The listing builds one solid part. Answer for the finished solid, in the listing's coordinates (mm). A direction names the side the tool comes from. Round coordinates to 2 decimals unless told otherwise and drop trailing zeros. Write each loop counter-clockwise with the first axis right and the second up, starting at its lowest first coordinate (ties: lowest second). Pieces come first, ordered by that corner, then holes. Notation, with made-up numbers: M 25,50.5 L 37,50.5 A12 ccw 37,59.5 Z; hole C 4,8.5 d9. An arc over 180 degrees is marked long. One line per item, written item: value. Start each with the question number.
(1) Given P1, Ø3, axis at x = -14, y = 0.5, coming from the +Z side; P2, Ø1.5, axis at x = 7.5, y = 2, coming from the -Z side; P3, Ø0.5, axis at x = -15, z = 0.5, coming from the -Y side, each flat-ended and moving along its own axis, determine where each tip first touches the part or whether it passes through.
(2) Section A-A (z = 0.6) is taken. Determine the outline of the cut face in (x, y) (3 decimals), plus the area to 3 significant figures.
(3) For a pull along X with two mould halves and no side action, classify faces 1 (the flat face through (0, -7, 1.092)), 2 (the flat face through (16.835, 7.3, 0.6)), 3 (the flat face through (9.835, 7.3, 0.6)) as released by +X, released by -X, zero draft, split by the parting line, or undercut.
(4) Consider probe 1 along X at (y, z) = (-8.5, 0.6); probe 2 along Y at (x, z) = (-14.5, 0.95) (3 decimals). Determine where each line is inside the solid, lowest interval first.
(5) Section C-C (x = 2.5) is taken. Determine the outline of the cut face in (y, z) (3 decimals).
(6) Section B-B (y = 7.5) is taken. Determine the outline of the cut face in (x, z).
(7) For faces 4 (the flat face through (-13.4, -5.123, 0.6)), 5 (the flat face through (-13.4, 9.525, 0.6)), 6 (the flat face through (13.3, -9.523, 0.6)), determine the directions among +Z, -Z, +X, -X, +Y, -Y from which every point of the face is accessible in a straight line to the end or side of a thin tool.
(8) Section D-D (x = 7) is taken. Determine the outline of the cut face in (y, z).
```python
from build123d import *

# Parameters (mm, degrees)
F0_W     = 41.0972
F0_H     = 25.4
F1_DEPTH = 0.0762
F2_W     = 7
F2_H     = 4.4
F3_DEPTH = 1.016
F4_DEPTH = 0.2032


with BuildPart() as f1:
    # F0 (on Top) → F1 (new body)
    with BuildSketch(Plane.XY):
        Rectangle(F0_W, F0_H)
    extrude(amount=F1_DEPTH)

    # F2 (on face) → F3 (join)
    with BuildSketch(Plane.XY.offset(0.0762)):
        with Locations((-13.33512, 7.325)):
            Rectangle(F2_W, F2_H)
        with Locations((-13.33512, -7.32318)):
            Rectangle(F2_W, F2_H)
        with Locations((-0.00012, 7.325)):
            Rectangle(F2_W, F2_H)
        with Locations((-0.00012, -7.32318)):
            Rectangle(F2_W, F2_H)
        with Locations((13.33488, 7.325)):
            Rectangle(F2_W, F2_H)
        with Locations((13.33488, -7.32318)):
            Rectangle(F2_W, F2_H)
    extrude(amount=F3_DEPTH)

    # F2 (on face) → F4 (join)
    with BuildSketch(Plane.XY.offset(0.0762)):
        with Locations((-13.33512, 7.325)):
            Rectangle(F2_W, F2_H)
        with Locations((-13.33512, -7.32318)):
            Rectangle(F2_W, F2_H)
        with Locations((-0.00012, 7.325)):
            Rectangle(F2_W, F2_H)
        with Locations((-0.00012, -7.32318)):
            Rectangle(F2_W, F2_H)
        with Locations((13.33488, 7.325)):
            Rectangle(F2_W, F2_H)
        with Locations((13.33488, -7.32318)):
            Rectangle(F2_W, F2_H)
    extrude(amount=-F4_DEPTH)


solid = f1.part
```
Recorded:
1. P1: stops at z = 0.08
1. P2: stops at z = 0
1. P3: stops at y = -9.52
2. outline: M -16.835,-9.523 L -9.835,-9.523 L -9.835,-5.123 L -16.835,-5.123 Z; M -16.835,5.125 L -9.835,5.125 L -9.835,9.525 L -16.835,9.525 Z; M -3.5,-9.523 L 3.5,-9.523 L 3.5,-5.123 L -3.5,-5.123 Z; M -3.5,5.125 L 3.5,5.125 L 3.5,9.525 L -3.5,9.525 Z; M 9.835,-9.523 L 16.835,-9.523 L 16.835,-5.123 L 9.835,-5.123 Z; M 9.835,5.125 L 16.835,5.125 L 16.835,9.525 L 9.835,9.525 Z
2. area: 185 mm2
3. face 1: zero draft
3. face 2: released by +X
3. face 3: undercut
4. probe 1: x = -16.84 to -9.84, -3.5 to 3.5, 9.83 to 16.83
4. probe 2: y = -9.523 to -5.123, 5.125 to 9.525
5. outline: M -12.7,0 L -9.523,0 L -9.523,-0.127 L -5.123,-0.127 L -5.123,0 L 5.125,0 L 5.125,-0.127 L 9.525,-0.127 L 9.525,0 L 12.7,0 L 12.7,0.076 L 9.525,0.076 L 9.525,1.092 L 5.125,1.092 L 5.125,0.076 L -5.123,0.076 L -5.123,1.092 L -9.523,1.092 L -9.523,0.076 L -12.7,0.076 Z
6. outline: M -20.55,0 L -16.84,0 L -16.84,-0.13 L -9.84,-0.13 L -9.84,0 L -3.5,0 L -3.5,-0.13 L 3.5,-0.13 L 3.5,0 L 9.83,0 L 9.83,-0.13 L 16.83,-0.13 L 16.83,0 L 20.55,0 L 20.55,0.08 L 16.83,0.08 L 16.83,1.09 L 9.83,1.09 L 9.83,0.08 L 3.5,0.08 L 3.5,1.09 L -3.5,1.09 L -3.5,0.08 L -9.84,0.08 L -9.84,1.09 L -16.84,1.09 L -16.84,0.08 L -20.55,0.08 Z
7. face 4: +Z, +X, -X
7. face 5: +Z, +X, -X, +Y
7. face 6: +Z, +X, -X, -Y
8. outline: M -12.7,0 L 12.7,0 L 12.7,0.08 L -12.7,0.08 Z
